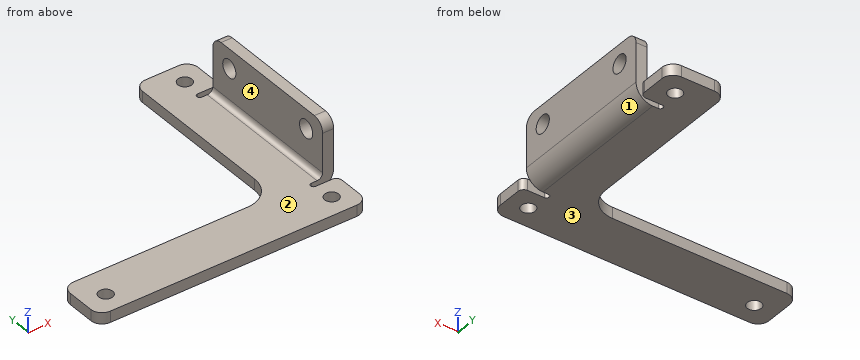
```python
from build123d import *

# Parameters (mm, degrees)
SKETCH1_W                 = 48.35
SKETCH1_H                 = 43.25
BOSS_EXTRUDE2_DEPTH       = 2
EDGE_FLANGE1_START        = -4
EDGE_FLANGE1_OUTLINE_W    = 1
EDGE_FLANGE1_OUTLINE_H    = 2
EDGE_FLANGE1_DEPTH        = 4
EDGE_FLANGE1_START_2      = -1
EDGE_FLANGE1_2_DEPTH      = 3.09178
EDGE_FLANGE1_START_3      = 2
EDGE_FLANGE1_3_OUTLINE_W  = 2
EDGE_FLANGE1_3_OUTLINE_H  = 26.65
EDGE_FLANGE1_3_DEPTH      = 10
EDGE_FLANGE1_START_4      = 8.3
EDGE_FLANGE1_4_DEPTH      = 26.65
EDGE_FLANGE1_5_DEPTH      = 26.65
EDGE_FLANGE1_START_5      = 46.35
EDGE_FLANGE1_6_OUTLINE_R  = 1.6
EDGE_FLANGE1_6_DEPTH      = 2
REDONDEO1_R               = 2
TALADRO_ROSCADO_M31_D     = 2.5
TALADRO_ROSCADO_M31_DEPTH = 8.5
TALADRO_ROSCADO_M31_TIP   = 0.751075774
CROQUIS4_W                = 38.35
CROQUIS4_H                = 34.25
CORTAR_EXTRUIR1_DEPTH     = 66.637527376
FILLET1_R                 = 2
REDONDEO2_R               = 5
REDONDEO3_R               = 1


with BuildPart() as part:
    # Sketch1 → Boss-Extrude2 (new body)
    with BuildSketch(Plane.XY):
        with Locations((24.175, 21.625)):
            Rectangle(SKETCH1_W, SKETCH1_H)
    extrude(amount=BOSS_EXTRUDE2_DEPTH)

    # Edge-Flange1: read off the stored shape, not the designer's step
    # Edge-Flange1 outline → Edge-Flange1 (cut)
    with BuildSketch(Plane(origin=(48.35, 0, 2), x_dir=(0, 1, 0), z_dir=(1, 0, 0)).offset(EDGE_FLANGE1_START)):
        with Locations((35.45, -1)):
            Rectangle(EDGE_FLANGE1_OUTLINE_W, EDGE_FLANGE1_OUTLINE_H)
        with Locations((7.8, -1)):
            Rectangle(EDGE_FLANGE1_OUTLINE_W, EDGE_FLANGE1_OUTLINE_H)
    extrude(amount=EDGE_FLANGE1_DEPTH, mode=Mode.SUBTRACT)

    # Edge-Flange1 2 outline → Edge-Flange1 2 (cut)
    with BuildSketch(Plane.XY.offset(EDGE_FLANGE1_START_2)):
        with BuildLine():
            Line((44.35, 7.3), (44.35, 8.3))
            ThreePointArc((44.35, 8.3), (43.85, 7.8), (44.35, 7.3))
        make_face()
        with BuildLine():
            ThreePointArc((44.35, 35.95), (43.85, 35.45), (44.35, 34.95))
            Line((44.35, 34.95), (44.35, 35.95))
        make_face()
    extrude(amount=EDGE_FLANGE1_2_DEPTH, mode=Mode.SUBTRACT)

    # Edge-Flange1 3 outline → Edge-Flange1 3 (add)
    with BuildSketch(Plane.XY.offset(EDGE_FLANGE1_START_3)):
        with Locations((47.35, 21.625)):
            Rectangle(EDGE_FLANGE1_3_OUTLINE_W, EDGE_FLANGE1_3_OUTLINE_H)
    extrude(amount=EDGE_FLANGE1_3_DEPTH)

    # Edge-Flange1 4 outline → Edge-Flange1 4 (add)
    with BuildSketch(Plane(origin=(0, 0, 0), x_dir=(1, 0, 0), z_dir=(0, 1, 0)).offset(EDGE_FLANGE1_START_4)):
        with BuildLine():
            Line((46.35, -3), (46.35, -2))
            Line((46.35, -2), (45.35, -2))
            ThreePointArc((45.35, -2), (46.057106781, -2.292893219), (46.35, -3))
        make_face()
    extrude(amount=EDGE_FLANGE1_4_DEPTH)

    # Edge-Flange1 5 outline → Edge-Flange1 5 (cut)
    with BuildSketch(Plane(origin=(0, 0, 0), x_dir=(1, 0, 0), z_dir=(0, 1, 0)).offset(EDGE_FLANGE1_START_4)):
        with BuildLine():
            Line((48.35, -3), (48.35, 0))
            Line((48.35, 0), (45.35, 0))
            ThreePointArc((45.35, 0), (47.471320344, -0.878679656), (48.35, -3))
        make_face()
    extrude(amount=EDGE_FLANGE1_5_DEPTH, mode=Mode.SUBTRACT)

    # Edge-Flange1 6 outline → Edge-Flange1 6 (cut)
    with BuildSketch(Plane.YZ.offset(EDGE_FLANGE1_START_5)):
        with Locations((12.3, 8.5)):
            Circle(EDGE_FLANGE1_6_OUTLINE_R)
        with Locations((30.95, 8.5)):
            Circle(EDGE_FLANGE1_6_OUTLINE_R)
    extrude(amount=EDGE_FLANGE1_6_DEPTH, mode=Mode.SUBTRACT)

    # Redondeo1
    redondeo1_edges = [part.edges().sort_by_distance(p)[0] for p in [
        (47.35, 8.3, 12),
        (47.35, 34.95, 12),
    ]]
    fillet(redondeo1_edges, radius=REDONDEO1_R)

    # Taladro roscado M31
    with Locations(Plane(origin=(0, 0, 0), x_dir=(-1, 0, 0), z_dir=(0, 0, -1))):
        with Locations((-44.65, 39.45), (-4, 3.8), (-44.65, 3.8)):
            Hole(TALADRO_ROSCADO_M31_D / 2, depth=TALADRO_ROSCADO_M31_DEPTH)
            with Locations((0, 0, -(TALADRO_ROSCADO_M31_DEPTH + TALADRO_ROSCADO_M31_TIP / 2))):  # 118° drill point
                Cone(0, TALADRO_ROSCADO_M31_D / 2, TALADRO_ROSCADO_M31_TIP, mode=Mode.SUBTRACT)

    # Croquis4 → Cortar-Extruir1 (cut, through all)
    with BuildSketch(Plane.XY.offset(2)):
        with Locations((19.175, 26.125)):
            Rectangle(CROQUIS4_W, CROQUIS4_H)
    extrude(amount=-CORTAR_EXTRUIR1_DEPTH, mode=Mode.SUBTRACT)

    # Fillet1
    fillet1_edges = [part.edges().sort_by_distance(p)[0] for p in [
        (0, 9, 1),
        (38.35, 43.25, 1),
        (0, 0, 1),
        (48.35, 43.25, 1),
        (48.35, 0, 1),
    ]]
    fillet(fillet1_edges, radius=FILLET1_R)

    # Redondeo2
    redondeo2_edges = [part.edges().sort_by_distance(p)[0] for p in [
        (38.35, 9, 1),
    ]]
    fillet(redondeo2_edges, radius=REDONDEO2_R)

    # Redondeo3
    redondeo3_edges = [part.edges().sort_by_distance(p)[0] for p in [
        (48.35, 35.95, 1),
        (48.35, 7.3, 1),
    ]]
    fillet(redondeo3_edges, radius=REDONDEO3_R)


solid = part.part
```
Geometry check sheet. Reference: the model listing, model coordinates, mm. Face numbers are marked on the shaded views. A direction names the side the tool comes from. Coordinates: 2 decimals unless noted, no trailing zeros. Order: outer loops, then holes, each group sorted by start corner. A loop starts at its lowest first (then second) coordinate and runs counter-clockwise, first axis right, second up.
Q1. Thickness scan on probe 1 along Y at (x, z) = (44.65, 1.65); probe 2 along Y at (x, z) = (4, 0.6); probe 3 along X at (y, z) = (19.5, 8.5). Record the ranges inside material, lowest first.
Reply:
probe 1: y = 0 to 2.55, 5.05 to 7.3, 8.3 to 34.95, 35.95 to 38.2, 40.7 to 43.25
probe 2: y = 0 to 2.55, 5.05 to 9
probe 3: x = 46.35 to 48.35
Q2. Draft check along Y on the marked faces 1 and 2. Enter one of: released by +Y, released by -Y, zero draft, split by the parting line, or undercut.
Reply:
face 1: undercut
face 2: zero draft
Q3. Sectioned sample at C-C on y = 3.8. Record the cut outline in (x, z), and give its area (3 significant figures).
Reply:
outline: (0, 0) - (2.75, 0) - (2.75, 2) - (0, 2) - close; (5.25, 0) - (43.4, 0) - (43.4, 2) - (5.25, 2) - close; (45.9, 0) - (48.35, 0) - (48.35, 2) - (45.9, 2) - close
area: 86.7 mm2
Q4. Sectioned sample at A-A on z = 8.5. Record the cut outline in (x, y).
Reply:
outline: (46.35, 8.3) - (48.35, 8.3) - (48.35, 10.7) - (46.35, 10.7) - close; (46.35, 13.9) - (48.35, 13.9) - (48.35, 29.35) - (46.35, 29.35) - close; (46.35, 32.55) - (48.35, 32.55) - (48.35, 34.95) - (46.35, 34.95) - close
Q5. Sectioned sample at D-D on y = 39.45. Record the cut outline in (x, z), and give its area (3 significant figures).
Reply:
outline: (38.35, 0) - (43.4, 0) - (43.4, 2) - (38.35, 2) - close; (45.9, 0) - (48.35, 0) - (48.35, 2) - (45.9, 2) - close
area: 15.0 mm2
Q6. Sectioned sample at B-B on x = 4. Record the cut outline in (y, z).
Reply:
outline: (0, 0) - (2.55, 0) - (2.55, 2) - (0, 2) - close; (5.05, 0) - (9, 0) - (9, 2) - (5.05, 2) - close
Q7. Depth check by flat-ended pin: pin 1 Ø0.6 at (x, z) = (20, 1) entering from +Y; pin 2 Ø1.5 at (y, z) = (34, 1.5) entering from -X; pin 3 Ø1.2 at (x, z) = (46.5, 6) entering from +Y. Enter the tip coordinate at first touch or a pass-through.
Reply:
pin 1: stops at y = 9
pin 2: stops at x = 38.35
pin 3: stops at y = 34.95
Q8. Tool access check on the marked faces 3 and 4. Record the directions out of +Z, -Z, +X, -X, +Y, -Y that give a thin tool (end or side, any length) a straight path to the whole face; none if there is none.
Reply:
face 3: -Z, +X, -X, +Y, -Y
face 4: +Z, -X, +Y, -Y
